from build123d import *

# Parameters (mm, degrees)
SKETCH1_W                  = 50
SKETCH1_H                  = 200
BOSS_EXTRUDE1_DEPTH        = 6
SKETCH2_W                  = 5.7
SKETCH2_H                  = 9
CUT_EXTRUDE1_DEPTH         = 6
CHAMFER2_SIZE              = 3
SKETCH3_W                  = 9
SKETCH3_H                  = 5.7
CUT_EXTRUDE2_DEPTH         = 10
CHAMFER3_SIZE              = 3
LPATTERN1_COUNT            = 10
LPATTERN1_PITCH            = 18
CHAMFER3_OF_LPATTERN1_SIZE = 3
MIRROR3_DEPTH              = 6


# Read off the part's stored shape, not the designer's step: Mirror3
with BuildPart() as part:
    # Sketch1 → Boss-Extrude1 (new body)
    with BuildSketch(Plane(origin=(0, 0, 0), x_dir=(1, 0, 0), z_dir=(0, 1, 0))):
        with Locations((25, 100)):
            Rectangle(SKETCH1_W, SKETCH1_H)
    extrude(amount=BOSS_EXTRUDE1_DEPTH)

    # Sketch2 → Cut-Extrude1 (cut)
    with BuildSketch(Plane(origin=(0, 6, 0), x_dir=(1, 0, 0), z_dir=(0, 1, 0))):
        with Locations((25, 195.5)):
            Rectangle(SKETCH2_W, SKETCH2_H)
        with Locations((25, 4.5)):
            Rectangle(SKETCH2_W, SKETCH2_H)
    extrude(amount=-CUT_EXTRUDE1_DEPTH, mode=Mode.SUBTRACT)

    # Chamfer2
    chamfer2_edges = [part.edges().sort_by_distance(p)[0] for p in [
        (22.15, 3, -200),
        (27.85, 3, -200),
        (27.85, 3, 0),
        (22.15, 3, 0),
    ]]
    chamfer(chamfer2_edges, length=CHAMFER2_SIZE)

    # Sketch3 → Cut-Extrude2 (cut)
    with BuildSketch(Plane(origin=(0, 6, 0), x_dir=(1, 0, 0), z_dir=(0, 1, 0))):
        with Locations((45.5, 182.15)):
            Rectangle(SKETCH3_W, SKETCH3_H)
    cut_extrude2 = extrude(amount=-CUT_EXTRUDE2_DEPTH, mode=Mode.SUBTRACT)

    # Chamfer3
    chamfer3_edges = [part.edges().sort_by_distance(p)[0] for p in [
        (50, 3, -185),
        (50, 3, -179.3),
    ]]
    chamfer(chamfer3_edges, length=CHAMFER3_SIZE)

    # LPattern1: Cut-Extrude2 ×10
    with Locations(*[(0, 0, i * LPATTERN1_PITCH) for i in range(1, LPATTERN1_COUNT)]):
        add(cut_extrude2, mode=Mode.SUBTRACT)

    # Chamfer3 of LPattern1
    chamfer3_of_lpattern1_edges = [part.edges().sort_by_distance(p)[0] for p in [
        (50, 3, -167),
        (50, 3, -161.3),
        (50, 3, -149),
        (50, 3, -143.3),
        (50, 3, -131),
        (50, 3, -125.3),
        (50, 3, -113),
        (50, 3, -107.3),
        (50, 3, -95),
        (50, 3, -89.3),
        (50, 3, -77),
        (50, 3, -71.3),
        (50, 3, -59),
        (50, 3, -53.3),
        (50, 3, -41),
        (50, 3, -35.3),
        (50, 3, -23),
        (50, 3, -17.3),
    ]]
    chamfer(chamfer3_of_lpattern1_edges, length=CHAMFER3_OF_LPATTERN1_SIZE)

    # Mirror3 outline → Mirror3 (cut)
    with BuildSketch(Plane(origin=(0, 0, 0), x_dir=(1, 0, 0), z_dir=(0, 1, 0))):
        Polygon((0, 176.3), (3, 179.3), (9, 179.3), (9, 185), (3, 185), (0, 188), align=None)
        Polygon((3, 23), (0, 26), (0, 14.3), (3, 17.3), (9, 17.3), (9, 23), align=None)
        Polygon((3, 41), (0, 44), (0, 32.3), (3, 35.3), (9, 35.3), (9, 41), align=None)
        Polygon((3, 59), (0, 62), (0, 50.3), (3, 53.3), (9, 53.3), (9, 59), align=None)
        Polygon((3, 77), (0, 80), (0, 68.3), (3, 71.3), (9, 71.3), (9, 77), align=None)
        Polygon((3, 95), (0, 98), (0, 86.3), (3, 89.3), (9, 89.3), (9, 95), align=None)
        Polygon((3, 113), (0, 116), (0, 104.3), (3, 107.3), (9, 107.3), (9, 113), align=None)
        Polygon((3, 131), (0, 134), (0, 122.3), (3, 125.3), (9, 125.3), (9, 131), align=None)
        Polygon((3, 149), (0, 152), (0, 140.3), (3, 143.3), (9, 143.3), (9, 149), align=None)
        Polygon((3, 167), (0, 170), (0, 158.3), (3, 161.3), (9, 161.3), (9, 167), align=None)
    extrude(amount=MIRROR3_DEPTH, mode=Mode.SUBTRACT)


solid = part.part
Design review of the part built by this model. Coordinates are the model's own, in mm. A direction names the side the tool comes from. Give positions to 0.01 mm unless a question says otherwise; leave off trailing zeros. Order: outer loops, then holes, each group sorted by start corner. A loop starts at its lowest first (then second) coordinate and runs counter-clockwise, first axis right, second up. Notation, with made-up numbers: (5.5, 24.5) - (21.5, 24.5) arc R9 ccw to (21.5, 38.5) - close; hole circle Ø10 at (67, 40). An arc over 180 degrees is marked (long way). Use CSV: the item, a comma, the result in double quotes. Start each with the question number.
Q1. Take a section at B-B (z = -19). State the section outline as (x, y) points, and give its area (3 significant figures).
Q2. For P1, Ø3, axis at y = 2.5, z = -19, coming from the +X side; P2, Ø3, axis at x = 24, y = 2.5, coming from the +Z side; P3, Ø1.5, axis at y = 5, z = -142, coming from the -X side; P4, Ø12, axis at x = 14.5, z = -136, coming from the -Y side, all flat-tipped, find the tip position at first contact; note any pin that passes through.
Q3. Draft analysis for pull direction Z (two halves, no side actions). For faces 4 (the face through (40, 3, -200)), 5 (the face through (9, 3, -38)), 6 (the face through (44, 3, -17.3)), 7 (the face through (50, 3, -47)), state which applies: pulls with the +Z half, pulls with the -Z half, needs draft (parallel to the pull), parting line crosses it, or undercut.
Q4. Take a section at A-A (x = 43). Count the separate pieces of the cut face and the enclosed holes in it, and give its area (3 significant figures).
Q5. Machinability: for faces 1 (the face through (50, 3, -194)), 2 (the face through (9, 3, -74)), 3 (the face through (41, 3, -92)), which of the approach directions +Z, -Z, +X, -X, +Y, -Y give a long, thin tool a straight path to every point of the face, cutting with its end or side? Answer none if there is none.
Q6. For line 1 (X direction, y = 1.3, z = -182); line 2 (Z direction, x = 28, y = 0.3); line 3 (X direction, y = 3.15, z = -150.5), list the stretches that pass through material, from the lowest coordinate up.
Calculated:
1,outline,"(9, 0) - (41, 0) - (41, 6) - (9, 6) - close"
1,area,"192 mm²"
2,P1,"stops at x = 41"
2,P2,"stops at z = -9"
2,P3,"stops at x = 0.95"
2,P4,"stops at y = 0"
3,face 4,"pulls with the -Z half"
3,face 5,"undercut"
3,face 6,"undercut"
3,face 7,"needs draft"
4,separate pieces,"11"
4,enclosed holes,"0"
4,area,"858 mm²"
5,face 1,"+Z, -Z, +X, +Y, -Y"
5,face 2,"-X, +Y, -Y"
5,face 3,"+X, +Y, -Y"
6,line 1,"x = 9 to 41"
6,line 2,"z = -197.15 to -2.85"
6,line 3,"x = 1.5 to 48.5"
